Design review of the part built by this model. Coordinates are the model's own, in mm. Face numbers are marked on the shaded views. A direction names the side the tool comes from. Coordinates: 2 decimals unless noted, no trailing zeros. Order: outer loops, then holes, each group sorted by start corner. A loop starts at its lowest first (then second) coordinate and runs counter-clockwise, first axis right, second up. Notation, with made-up numbers: (-34.5, 61.25) -> (11.5, 61.25) arc R16 cw to (11.5, 72.25) -> close; hole circle Ø8 at (-15.5, -30.75). An arc over 180 degrees is marked (long way). Use a Markdown table: item, result. Add a question column.
Q1. Add section C-C (y = 4). State the section outline as (x, z) points, then the cut area to 3 significant figures.
Q2. Machinability: for the marked faces 1 and 2, which of the approach directions +Z, -Z, +X, -X, +Y, -Y give a long, thin tool a straight path to every point of the face, cutting with its end or side? Answer none if there is none.
Q3. Wall thickness on probe 1 along X at (y, z) = (0, 9.25); probe 2 along Y at (x, z) = (0, 2.3) (3 decimals): over which ranges is each line inside the solid? List them lowest first.
Q4. Insertion check: pin 1 (2 mm diameter, centred on x = 0, y = 0, fed in from -Z); pin 2 (1.8 mm diameter, centred on x = 0, y = -0.5, fed in from +Z); pin 3 (1.5 mm diameter, centred on y = -0.5, z = 11.5, fed in from +X); pin 4 (1 mm diameter, centred on y = 1, z = 19.5, fed in from +X). Each pin has a flat end and moves straight along its axis. Give the tip position at first contact, or say it passes through.
Q5. The part is to be moulded in two halves that separate along X. For the marked faces 3, 4 and 5, say which applies: pulls with the +X half, pulls with the -X half, needs draft (parallel to the pull), parting line crosses it, or undercut.
Q6. Add section D-D (x = -2.25). State the section outline as (y, z) points.
Q7. Add section B-B (z = 18). State the section outline as (x, y) points, then the cut area to 3 significant figures.
from build123d import *

# Parameters (mm, degrees)
CROQUIS1_R                 = 2.5
CROQUIS1_R_2               = 1.8
SALIENTE_EXTRUIR1_DEPTH    = 24
CROQUIS3_R                 = 1.8
SALIENTE_EXTRUIR2_DEPTH    = 3.15
CORTAR_EXTRUIR1_DEPTH      = 25.259018941
CORTAR_EXTRUIR1_DEPTH_BACK = 25.259018941
CROQUIS4_R                 = 1.265
CROQUIS5_R                 = 5
CROQUIS5_R_2               = 1.8
SALIENTE_EXTRUIR3_DEPTH    = 1.5


with BuildPart() as part:
    # Croquis1 → Saliente-Extruir1 (new body)
    with BuildSketch(Plane.XY):
        Circle(CROQUIS1_R)
        Circle(CROQUIS1_R_2, mode=Mode.SUBTRACT)
    extrude(amount=SALIENTE_EXTRUIR1_DEPTH)

    # Croquis3 → Saliente-Extruir2 (add)
    with BuildSketch(Plane(origin=(0, 0, 0), x_dir=(-1, 0, 0), z_dir=(0, 0, -1))):
        Circle(CROQUIS3_R)
    extrude(amount=-SALIENTE_EXTRUIR2_DEPTH)

    # Croquis4 → Cortar-Extruir1 (cut, two sides: drawn at the far end of the back side and taken through both)
    with BuildSketch(Plane(origin=(0, 0, 0), x_dir=(-1, 0, 0), z_dir=(0, 0, -1)).offset(-CORTAR_EXTRUIR1_DEPTH_BACK)):
        Circle(CROQUIS4_R)
    extrude(amount=CORTAR_EXTRUIR1_DEPTH + CORTAR_EXTRUIR1_DEPTH_BACK, mode=Mode.SUBTRACT)

    # Croquis5 → Saliente-Extruir3 (add, symmetric)
    with BuildSketch(Plane.XY.offset(24)):
        Circle(CROQUIS5_R)
        with Locations(Location((0, 0, 0), (0, 0, 180))):
            Circle(CROQUIS5_R_2, mode=Mode.SUBTRACT)
    extrude(amount=SALIENTE_EXTRUIR3_DEPTH, both=True)


solid = part.part
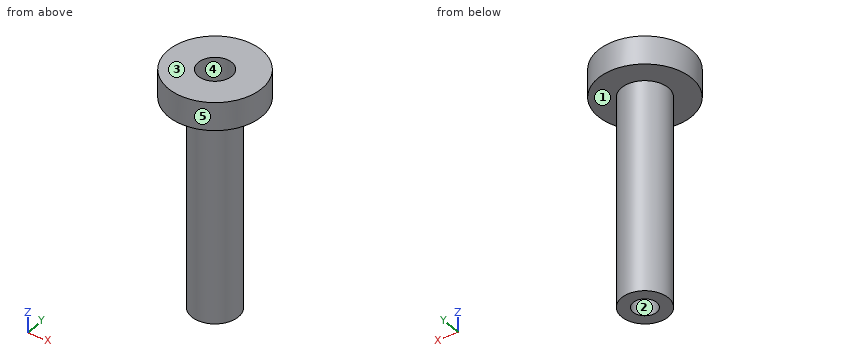
Established:
| question | item | result |
|---|---|---|
| 1 | outline | (-3, 22.5) -> (3, 22.5) -> (3, 25.5) -> (-3, 25.5) -> close |
| 1 | area | 18.0 mm^2 |
| 2 | face 1 | -Z |
| 2 | face 2 | +Z, -Z |
| 3 | probe 1 | -2.5 to -1.8, 1.8 to 2.5 |
| 3 | probe 2 | -2.5 to -1.265, 1.265 to 2.5 |
| 4 | pin 1 | through |
| 4 | pin 2 | z = 3.15 |
| 4 | pin 3 | x = 2.5 |
| 4 | pin 4 | x = 2.45 |
| 5 | face 3 | needs draft |
| 5 | face 4 | undercut |
| 5 | face 5 | parting line crosses it |
| 6 | outline | (-4.47, 22.5) -> (-1.09, 22.5) -> (-1.09, 0) -> (1.09, 0) -> (1.09, 22.5) -> (4.47, 22.5) -> (4.47, 25.5) -> (-4.47, 25.5) -> close |
| 7 | outline | circle Ø5 at (0, 0); hole circle Ø3.6 at (0, 0) |
| 7 | area | 9.46 mm^2 |
